Here's how the part is built. I have some questions about the finished solid (model axes, mm). Give positions to 0.01 mm unless a question says otherwise; leave off trailing zeros. Order: outer loops, then holes, each group sorted by start corner. A loop starts at its lowest first (then second) coordinate and runs counter-clockwise, first axis right, second up. Notation, with made-up numbers: M 70.25,-29 L 118.25,-29 A21 ccw 118.25,-13 Z; hole C 12.5,-33 d3. An arc over 180 degrees is marked long. Use one line per item in the form item = value.
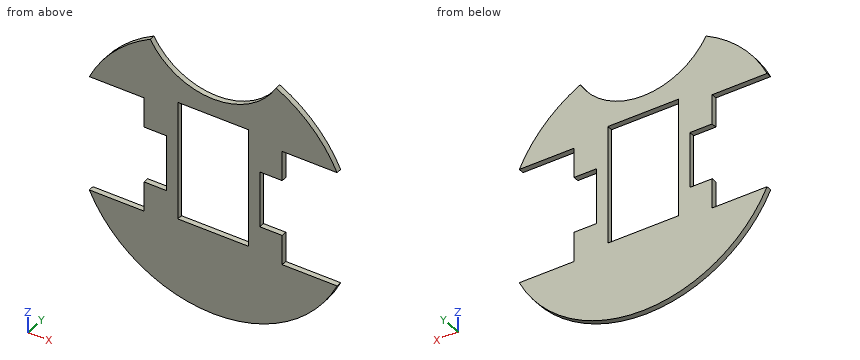
from build123d import *

# Parameters (mm, degrees)
BOSS_EXTRUDE1_DEPTH  = 2.9
SOLENOID_PLACEMENT_W = 37.4
SOLENOID_PLACEMENT_H = 63.8
CUT_EXTRUDE1_DEPTH   = 103.571487266
CUT_EXTRUDE2_DEPTH   = 103.571487266


with BuildPart() as part:
    # Sketch1 → Boss-Extrude1 (new body)
    with BuildSketch(Plane(origin=(0, 0, 0), x_dir=(1, 0, 0), z_dir=(0, 1, 0))):
        with BuildLine():
            ThreePointArc((33.29110537, -64.404598464), (0, 72.5), (-33.29110537, -64.404598464))
            ThreePointArc((-33.29110537, -64.404598464), (0, -44.989799638), (33.29110537, -64.404598464))
        make_face()
    extrude(amount=BOSS_EXTRUDE1_DEPTH)

    # solenoid placement → Cut-Extrude1 (cut, through all)
    with BuildSketch(Plane(origin=(0, 2.9, 0), x_dir=(1, 0, 0), z_dir=(0, 1, 0))):
        with Locations((0, -3.8)):
            Rectangle(SOLENOID_PLACEMENT_W, SOLENOID_PLACEMENT_H)
    extrude(amount=-CUT_EXTRUDE1_DEPTH, mode=Mode.SUBTRACT)

    # Sketch2 → Cut-Extrude2 (cut, through all)
    with BuildSketch(Plane(origin=(0, 2.9, 0), x_dir=(1, 0, 0), z_dir=(0, 1, 0))):
        with BuildLine():
            Line((-36.51, -15), (-24.71, -15))
            Line((-24.71, -15), (-24.71, 15))
            Line((-24.71, 15), (-36.51, 15))
            Line((-36.51, 15), (-36.51, 31))
            Line((-36.51, 31), (-65.538156825, 31))
            ThreePointArc((-65.538156825, 31), (-72.5, 0), (-65.538156825, -31))
            Line((-65.538156825, -31), (-36.51, -31))
            Line((-36.51, -31), (-36.51, -15))
        make_face()
        with BuildLine():
            Line((36.51, -31), (65.538156825, -31))
            ThreePointArc((65.538156825, -31), (72.5, 0), (65.538156825, 31))
            Line((65.538156825, 31), (36.51, 31))
            Line((36.51, 31), (36.51, 15))
            Line((36.51, 15), (24.71, 15))
            Line((24.71, 15), (24.71, -15))
            Line((24.71, -15), (36.51, -15))
            Line((36.51, -15), (36.51, -31))
        make_face()
    extrude(amount=-CUT_EXTRUDE2_DEPTH, mode=Mode.SUBTRACT)


solid = part.part
Q1. I want a section at D-D on z = -58. Write out the boundary of the cut face in (x, y).
Found:
outline = M -43.5,0 L 43.5,0 L 43.5,2.9 L -43.5,2.9 Z
Q2. I need wall thicknesses on L1, parallel to X at y = 1.1, z = -12.5; L2, parallel to X at y = 1.65, z = 27.5; L3, parallel to Z at x = 35, y = 0.9. Which ranges of each line are inside material? Lowest first, please.
Found:
L1 = -24.71 to -18.7, 18.7 to 24.71
L2 = -36.51 to -18.7, 18.7 to 36.51
L3 = -63.49 to -15, 15 to 63.49
Q3. I'm going to push flat-ended pins straight in: pin 1 Ø0.9 at (x, y) = (-29, 1.5) entering from +Z; pin 2 Ø1.4 at (x, y) = (-56, 1) entering from +Z; pin 3 Ø0.9 at (x, y) = (32, 1) entering from -Z; pin 4 Ø8 at (x, z) = (-49, -28) entering from +Y. Where does each tip first touch, or does it pass through?
Found:
pin_1 = 58.83
pin_2 = 46.88
pin_3 = -65.28
pin_4 = 2.9
Q4. I want a section at C-C on x = -3. Write out the boundary of the cut face in (y, z).
Found:
outline = M 0,-72.44 L 2.9,-72.44 L 2.9,-28.1 L 0,-28.1 Z; M 0,35.7 L 2.9,35.7 L 2.9,45.11 L 0,45.11 Z
Q5. I want a section at B-B on y = 1.6. Write out the boundary of the cut face in (x, z).
Found:
outline = M -65.54,-31 A72.5 ccw 65.54,-31 L 36.51,-31 L 36.51,-15 L 24.71,-15 L 24.71,15 L 36.51,15 L 36.51,31 L 65.54,31 A72.5 ccw 33.29,64.4 A38.25 cw -33.29,64.4 A72.5 ccw -65.54,31 L -36.51,31 L -36.51,15 L -24.71,15 L -24.71,-15 L -36.51,-15 L -36.51,-31 Z; hole M -18.7,-28.1 L 18.7,-28.1 L 18.7,35.7 L -18.7,35.7 Z
Q6. I want a section at A-A on z = -1. Write out the boundary of the cut face in (x, y).
Found:
outline = M -24.71,0 L -18.7,0 L -18.7,2.9 L -24.71,2.9 Z; M 18.7,0 L 24.71,0 L 24.71,2.9 L 18.7,2.9 Z
